from build123d import *

# Parameters (mm, degrees)
F1_DEPTH = 76.2
F2_W     = 4.913513
F2_H     = 76.708
F3_DEPTH = 50.8


with BuildPart() as f1:
    # F0 (on Top) → F1 (new body, symmetric)
    with BuildSketch(Plane.XY):
        with BuildLine():
            Line((-14.237757, -4.885755), (-19.169552, -4.935114))
            ThreePointArc((-19.169552, -4.935114), (-31.159886, -46.375263), (-23.097479, -88.755114))
            Line((-23.097479, -88.755114), (-17.844147, -89.975755))
            ThreePointArc((-17.844147, -89.975755), (-26.952715, -46.96828), (-14.237757, -4.885755))
        make_face()
    extrude(amount=F1_DEPTH, both=True)

    # F2 (on Right) → F3 (cut)
    with BuildSketch(Plane.YZ):
        with Locations((-54.332511, 0)):
            Rectangle(F2_W, F2_H)
    extrude(amount=-F3_DEPTH, mode=Mode.SUBTRACT)


solid = f1.part
Work out the finished part from the listing and answer in its coordinate system (mm). A direction names the side the tool comes from. Give positions to 0.01 mm unless a question says otherwise; leave off trailing zeros. Order: outer loops, then holes, each group sorted by start corner. A loop starts at its lowest first (then second) coordinate and runs counter-clockwise, first axis right, second up. Notation, with made-up numbers: (21.5, 4) - (44.5, 4) arc R25 ccw to (44.5, 41) - close; hole circle Ø6 at (-0.5, -30.75). An arc over 180 degrees is marked (long way). Answer as CSV lines item,"result". Start each with the question number.
Q1. The part is cut by section A-A (z = -33). Write down the section's boundary in (x, y), then the cut area to 3 significant figures.
Q2. Find the intervals of material crossed by L1, parallel to Y at x = -19.5, z = 20; L2, parallel to X at y = -56.5, z = -46; L3, parallel to X at y = -67, z = -66, in increasing order. Write a range as [from, to].
Q3. The part is cut by section B-B (x = -21). Write down the section's boundary in (y, z).
Q4. The mould has two halves that part along Z. Classify faces 3 (the face through (-27, -44, 76.2)), 4 (the face through (-29, -51.876, -1)), 5 (the face through (-20.508, -89.357, 1.067)): +Z half, -Z half, draft (parallel to the pull), parting line (faces both ways), or undercut.
Q5. The part is cut by section C-C (y = -68). Write down the section's boundary in (x, z), then the cut area to 3 significant figures.
Q6. Given pin 1 Ø12 at (y, z) = (-58.5, 53.5) entering from +X; pin 2 Ø2 at (x, z) = (-20.5, -28) entering from +Y, each flat-ended and moving along its own axis, determine where each tip first touches the part or whether it passes through.
Q7. The part is cut by section D-D (z = 46.5). Write down the section's boundary in (x, y).
Q8. For faces 1 (the face through (-26.977, -47.59, 1.067)), 2 (the face through (-29, -56.789, -1)), determine the directions among +Z, -Z, +X, -X, +Y, -Y from which every point of the face is accessible in a straight line to the end or side of a thin tool.
Check result:
1,outline,"(-31.25, -51.88) - (-27.02, -51.88) arc R88.48 cw to (-14.24, -4.89) - (-19.17, -4.94) arc R92.71 ccw to start; (-31.06, -56.79) arc R92.71 ccw to (-23.1, -88.76) - (-17.84, -89.98) arc R88.48 cw to (-26.82, -56.79) - close"
1,area,"351 mm²"
2,L1,"y = [-89.59, -86.44], [-14.99, -5.52]"
2,L2,"x = [-31.08, -26.84]"
2,L3,"x = [-29.82, -25.52]"
3,outline,"(-89.24, -76.2) - (-82.82, -76.2) - (-82.82, 76.2) - (-89.24, 76.2) - close; (-18.61, -76.2) - (-8.32, -76.2) - (-8.32, 76.2) - (-18.61, 76.2) - close"
4,face 3,"+Z half"
4,face 4,"undercut"
4,face 5,"draft"
5,outline,"(-29.64, -76.2) - (-25.33, -76.2) - (-25.33, 76.2) - (-29.64, 76.2) - close"
5,area,"657 mm²"
6,pin 1,"stops at x = -25.95"
6,pin 2,"stops at y = -5.52"
7,outline,"(-23.1, -88.76) - (-17.84, -89.98) arc R88.48 cw to (-14.24, -4.89) - (-19.17, -4.94) arc R92.71 ccw to start"
8,face 1,"+Z, -Z, +X"
8,face 2,"+X, -X"
